Work out the finished part from the listing and answer in its coordinate system (mm). A direction names the side the tool comes from. Give positions to 0.01 mm unless a question says otherwise; leave off trailing zeros. Use one line per item in the form item = value. Start each with the question number.
from build123d import *

# Parameters (mm, degrees)
F0_R     = 2.1
F1_DEPTH = 200
F2_R     = 2.1
F3_DEPTH = 7


with BuildPart() as f1:
    # F0 (on Top) → F1 (new body)
    with BuildSketch(Plane.XY):
        with BuildLine():
            ThreePointArc((-3.308023, 10.226634), (-3.381246, 10.403411), (-3.558023, 10.476634))
            Line((-3.558023, 10.476634), (-10.308023, 10.476634))
            ThreePointArc((-10.308023, 10.476634), (-10.499365, 10.438574), (-10.661577, 10.330188))
            ThreePointArc((-10.661577, 10.330188), (-10.769963, 10.167976), (-10.808023, 9.976634))
            Line((-10.808023, 9.976634), (-10.808023, 3.226634))
            ThreePointArc((-10.808023, 3.226634), (-10.7348, 3.049858), (-10.558023, 2.976634))
            Line((-10.558023, 2.976634), (-9.555049, 2.976634))
            ThreePointArc((-9.555049, 2.976634), (-9.378272, 3.049858), (-9.305049, 3.226634))
            Line((-9.305049, 3.226634), (-9.305049, 6.654412))
            ThreePointArc((-9.305049, 6.654412), (-9.024273, 7.159685), (-8.45447, 7.062421))
            Line((-8.45447, 7.062421), (-4.381246, 2.989198))
            ThreePointArc((-4.381246, 2.989198), (-4.327053, 2.908092), (-4.308023, 2.812421))
            Line((-4.308023, 2.812421), (-4.308023, -1.859152))
            ThreePointArc((-4.308023, -1.859152), (-4.327053, -1.954823), (-4.381246, -2.035929))
            Line((-4.381246, -2.035929), (-8.45447, -6.109152))
            ThreePointArc((-8.45447, -6.109152), (-8.999365, -6.217538), (-9.308023, -5.755599))
            Line((-9.308023, -5.755599), (-9.308023, -2.273366))
            ThreePointArc((-9.308023, -2.273366), (-9.381246, -2.096589), (-9.558023, -2.023366))
            Line((-9.558023, -2.023366), (-10.558023, -2.023366))
            ThreePointArc((-10.558023, -2.023366), (-10.7348, -2.096589), (-10.808023, -2.273366))
            Line((-10.808023, -2.273366), (-10.808023, -9.023366))
            ThreePointArc((-10.808023, -9.023366), (-10.769963, -9.214707), (-10.661577, -9.376919))
            ThreePointArc((-10.661577, -9.376919), (-10.508248, -9.481525), (-10.327327, -9.522993))
            Line((-10.327327, -9.522993), (-3.544376, -9.522993))
            ThreePointArc((-3.544376, -9.522993), (-3.376486, -9.44525), (-3.308023, -9.273366))
            Line((-3.308023, -9.273366), (-3.308023, -8.273366))
            ThreePointArc((-3.308023, -8.273366), (-3.381246, -8.096589), (-3.558023, -8.023366))
            Line((-3.558023, -8.023366), (-7.040256, -8.023366))
            ThreePointArc((-7.040256, -8.023366), (-7.502196, -7.714707), (-7.39381, -7.169812))
            Line((-7.39381, -7.169812), (-3.320586, -3.096589))
            ThreePointArc((-3.320586, -3.096589), (-3.23948, -3.042396), (-3.14381, -3.023366))
            Line((-3.14381, -3.023366), (1.527763, -3.023366))
            ThreePointArc((1.527763, -3.023366), (1.623434, -3.042396), (1.70454, -3.096589))
            Line((1.70454, -3.096589), (5.777763, -7.169812))
            ThreePointArc((5.777763, -7.169812), (5.88615, -7.714707), (5.42421, -8.023366))
            Line((5.42421, -8.023366), (1.95454, -8.023366))
            ThreePointArc((1.95454, -8.023366), (1.777763, -8.096589), (1.70454, -8.273366))
            Line((1.70454, -8.273366), (1.70454, -9.273366))
            ThreePointArc((1.70454, -9.273366), (1.773002, -9.44525), (1.940893, -9.522993))
            Line((1.940893, -9.522993), (8.711281, -9.522993))
            ThreePointArc((8.711281, -9.522993), (8.892202, -9.481525), (9.04553, -9.376919))
            ThreePointArc((9.04553, -9.376919), (9.141878, -9.241515), (9.188525, -9.082012))
            Line((9.188525, -9.082012), (9.188525, -2.231968))
            ThreePointArc((9.188525, -2.231968), (9.103455, -2.082513), (8.941977, -2.023366))
            Line((8.941977, -2.023366), (7.941977, -2.023366))
            ThreePointArc((7.941977, -2.023366), (7.7652, -2.096589), (7.691977, -2.273366))
            Line((7.691977, -2.273366), (7.691977, -5.755599))
            ThreePointArc((7.691977, -5.755599), (7.383319, -6.217538), (6.838423, -6.109152))
            Line((6.838423, -6.109152), (2.7652, -2.035929))
            ThreePointArc((2.7652, -2.035929), (2.711007, -1.954823), (2.691977, -1.859152))
            Line((2.691977, -1.859152), (2.691977, 2.812421))
            ThreePointArc((2.691977, 2.812421), (2.711007, 2.908092), (2.7652, 2.989198))
            Line((2.7652, 2.989198), (6.838423, 7.062421))
            ThreePointArc((6.838423, 7.062421), (7.383319, 7.170807), (7.691977, 6.708867))
            Line((7.691977, 6.708867), (7.691977, 3.226634))
            ThreePointArc((7.691977, 3.226634), (7.7652, 3.049858), (7.941977, 2.976634))
            Line((7.941977, 2.976634), (8.941977, 2.976634))
            ThreePointArc((8.941977, 2.976634), (9.103455, 3.035782), (9.188525, 3.185237))
            Line((9.188525, 3.185237), (9.188525, 10.035281))
            ThreePointArc((9.188525, 10.035281), (9.141878, 10.194784), (9.04553, 10.330188))
            ThreePointArc((9.04553, 10.330188), (8.883319, 10.438574), (8.691977, 10.476634))
            Line((8.691977, 10.476634), (1.941977, 10.476634))
            ThreePointArc((1.941977, 10.476634), (1.7652, 10.403411), (1.691977, 10.226634))
            Line((1.691977, 10.226634), (1.691977, 9.226634))
            ThreePointArc((1.691977, 9.226634), (1.695138, 9.187006), (1.70454, 9.14838))
            ThreePointArc((1.70454, 9.14838), (1.795456, 9.024071), (1.941977, 8.976634))
            Line((1.941977, 8.976634), (5.42421, 8.976634))
            ThreePointArc((5.42421, 8.976634), (5.88615, 8.667976), (5.777763, 8.123081))
            Line((5.777763, 8.123081), (1.70454, 4.049858))
            ThreePointArc((1.70454, 4.049858), (1.623434, 3.995664), (1.527763, 3.976634))
            Line((1.527763, 3.976634), (-3.14381, 3.976634))
            ThreePointArc((-3.14381, 3.976634), (-3.23948, 3.995664), (-3.320586, 4.049858))
            Line((-3.320586, 4.049858), (-7.39381, 8.123081))
            ThreePointArc((-7.39381, 8.123081), (-7.502196, 8.667976), (-7.040256, 8.976634))
            Line((-7.040256, 8.976634), (-3.558023, 8.976634))
            ThreePointArc((-3.558023, 8.976634), (-3.381246, 9.049858), (-3.308023, 9.226634))
            Line((-3.308023, 9.226634), (-3.308023, 9.726634))
            Line((-3.308023, 9.726634), (-3.308023, 10.226634))
        make_face()
        with Locations((-0.808023, 0.476634)):
            Circle(F0_R, mode=Mode.SUBTRACT)
    extrude(amount=F1_DEPTH)

    # F2 (on face) → F3 (cut)
    with BuildSketch(Plane.YZ.offset(2.691977)):
        with Locations((0.476634, 79.99858)):
            Circle(F2_R)
    extrude(amount=-F3_DEPTH, mode=Mode.SUBTRACT)


solid = f1.part
1) Flat-ended cylindrical pins translate along their axes: pin 1 Ø1.4 at (x, z) = (0, 55.5) entering from -Y; pin 2 Ø1.4 at (y, z) = (0.5, 126.5) entering from +X; pin 3 Ø10 at (x, y) = (-1.5, -3.5) entering from -Z; pin 4 Ø1.4 at (x, z) = (-0.5, 97) entering from +Y. Find the tip coordinate at first contact, or state that the pin passes through.
2) Find the intervals of material crossed by probe 1 along X at (y, z) = (-5.75, 139.5); probe 2 along Y at (x, z) = (-5.25, 140); probe 3 along Y at (x, z) = (-6.5, 28.5), in increasing order.
3) Determine the mould class of faces 4 (the flat face through (9.189, -6, 99)), 5 (the cylindrical face through (-2.92, -1.19, 78.72)), 6 (the flat face through (-1, -3.023, 99)) for opening direction Y: released by +Y, released by -Y, zero draft, split by the parting line, or undercut.
4) A tool of negligible diameter and unlimited length cuts with its end or side. For faces 1 (the flat face through (4.773, 4.997, 98.6)), 2 (the flat face through (-4.308, 1, 99)), 3 (the flat face through (-1, 3.977, 99)), from which of +Z, -Z, +X, -X, +Y, -Y can it reach the whole face along a straight path? Write none if from no direction.
Answer sheet:
q1.pin_1 = -3.02
q1.pin_2 = 2.69
q1.pin_3 = 0
q1.pin_4 = 3.98
q2.probe_1 = -10.81 to -9.31, -8.1 to -5.97, 4.36 to 6.48, 7.69 to 9.19
q2.probe_2 = -9.52 to -8.02, -5.03 to -2.9, 3.86 to 5.98, 8.98 to 10.48
q2.probe_3 = -9.52 to -8.02, -6.28 to -4.15, 5.11 to 7.23, 8.98 to 10.48
q3.face_4 = zero draft
q3.face_5 = undercut
q3.face_6 = released by -Y
q4.face_1 = +Z, -Z
q4.face_2 = +Z, -Z, -X
q4.face_3 = +Z, -Z, +Y
